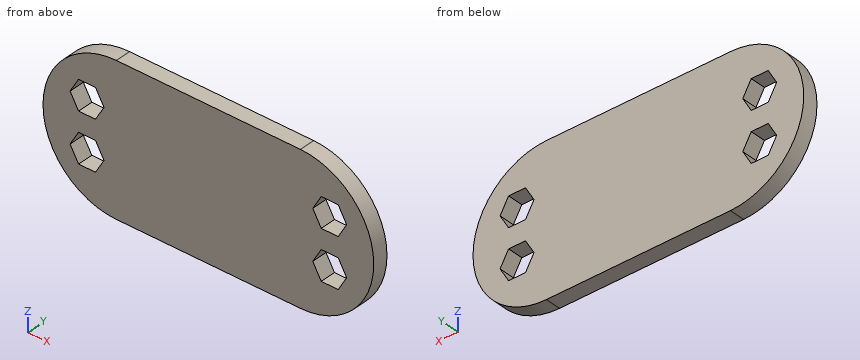
from build123d import *

# Parameters (mm, degrees)
BOSS_EXTRUDE1_DEPTH = 3.175


with BuildPart() as part:
    # Sketch2 → Boss-Extrude1 (new body)
    with BuildSketch(Plane(origin=(0, 0, 0), x_dir=(1, 0, 0), z_dir=(0, 1, 0))):
        with BuildLine():
            Line((-145.521414695, 0.997059393), (-107.921414695, 0.997059393))
            ThreePointArc((-107.921414695, 0.997059393), (-92.921414695, -14.002940607), (-107.921414695, -29.002940607))
            Line((-107.921414695, -29.002940607), (-145.521414695, -29.002940607))
            ThreePointArc((-145.521414695, -29.002940607), (-160.521414695, -14.002940607), (-145.521414695, 0.997059393))
        make_face()
        Polygon((-149.789363887, -12.002940607), (-148.05731308, -9.002940607), (-149.789363887, -6.002940607), (-153.253465503, -6.002940607), (-154.98551631, -9.002940607), (-153.253465503, -12.002940607), align=None, mode=Mode.SUBTRACT)
        Polygon((-153.253465503, -16.002940607), (-149.789363887, -16.002940607), (-148.05731308, -19.002940607), (-149.789363887, -22.002940607), (-153.253465503, -22.002940607), (-154.98551631, -19.002940607), align=None, mode=Mode.SUBTRACT)
        Polygon((-103.653465503, -16.002940607), (-105.38551631, -19.002940607), (-103.653465503, -22.002940607), (-100.189363887, -22.002940607), (-98.45731308, -19.002940607), (-100.189363887, -16.002940607), align=None, mode=Mode.SUBTRACT)
        Polygon((-100.189363887, -12.002940607), (-103.653465503, -12.002940607), (-105.38551631, -9.002940607), (-103.653465503, -6.002940607), (-100.189363887, -6.002940607), (-98.45731308, -9.002940607), align=None, mode=Mode.SUBTRACT)
    extrude(amount=BOSS_EXTRUDE1_DEPTH)


solid = part.part
Read the model definition and answer for the solid it produces. Units are mm, in the model's axes. Coordinates: 2 decimals unless noted, no trailing zeros. Loops run counter-clockwise (first coordinate to the right, second up) from the corner with the lowest first, then second, coordinate; pieces in that order, holes last. Notation, with made-up numbers: (-16, 86) -> (10, 86) arc R35 cw to (10, 125) -> close; hole circle Ø2 at (14, 13). An arc over 180 degrees is marked (long way). Answer in a Markdown table with one row per item.
Item 1: Each of these flat-tipped pins is pushed along its axis until it touches: P1, Ø1, axis at x = -102, y = 2, coming from the -Z side; P2, Ø1.6, axis at x = -101, y = 1.5, coming from the -Z side; P3, Ø1.6, axis at x = -101.5, y = 1.5, coming from the +Z side. Where does it stop, or does it pass through?
Returned:
| item | result |
|---|---|
| P1 | stops at z = 0.02 |
| P2 | stops at z = 0.31 |
| P3 | stops at z = 27.91 |
Item 2: A cutting plane is placed at C-C on z = 27. Determine the outline of the cut face in (x, y) (3 decimals).
Returned:
| item | result |
|---|---|
| outline | (-153.01, 0) -> (-100.433, 0) -> (-100.433, 3.175) -> (-153.01, 3.175) -> close |
Item 3: A cutting plane is placed at A-A on y = 2.3. Determine the outline of the cut face in (x, z), plus the area to 3 significant figures.
Returned:
| item | result |
|---|---|
| outline | (-145.52, -1) -> (-107.92, -1) arc R15 ccw to (-107.92, 29) -> (-145.52, 29) arc R15 ccw to start; hole (-154.99, 9) -> (-153.25, 6) -> (-149.79, 6) -> (-148.06, 9) -> (-149.79, 12) -> (-153.25, 12) -> close; hole (-154.99, 19) -> (-153.25, 16) -> (-149.79, 16) -> (-148.06, 19) -> (-149.79, 22) -> (-153.25, 22) -> close; hole (-105.39, 9) -> (-103.65, 6) -> (-100.19, 6) -> (-98.46, 9) -> (-100.19, 12) -> (-103.65, 12) -> close; hole (-105.39, 19) -> (-103.65, 16) -> (-100.19, 16) -> (-98.46, 19) -> (-100.19, 22) -> (-103.65, 22) -> close |
| area | 1,710 mm^2 |
Item 4: Straight lines are drawn through the part: line 1 along Z through (x, y) = (-149.5, 2.9); line 2 along Z through (x, y) = (-153, 0.85); line 3 along X through (y, z) = (0.85, 21). For each, find the intervals that lie inside material, in ascending order. Write a range as [from, to].
Returned:
| item | result |
|---|---|
| line 1 | z = [-0.46, 6.5], [11.5, 16.5], [21.5, 28.47] |
| line 2 | z = [1, 6], [12, 16], [22, 27.01] |
| line 3 | x = [-158.79, -153.83], [-149.21, -104.23], [-99.61, -94.65] |
Item 5: A cutting plane is placed at B-B on z = 7.75. Determine the outline of the cut face in (x, y) (3 decimals).
Returned:
| item | result |
|---|---|
| outline | (-159.156, 0) -> (-154.262, 0) -> (-154.262, 3.175) -> (-159.156, 3.175) -> close; (-148.781, 0) -> (-104.662, 0) -> (-104.662, 3.175) -> (-148.781, 3.175) -> close; (-99.181, 0) -> (-94.287, 0) -> (-94.287, 3.175) -> (-99.181, 3.175) -> close |
